Input: part model. Units: mm. Frame: model coordinates. Coordinates: 2 decimals unless noted, no trailing zeros. Use CSV: the item, a comma, the result in double quotes.
```python
from build123d import *

# Parameters (mm, degrees)
F0_R     = 19.05
F1_DEPTH = 6.35
F2_D     = 6.7564
F2_DEPTH = 6.35
F2_TIP   = 2.0298273432


# Not quite as in the source:
# - ends of sketch curves that miss each other by under 0.0002 mm in the source are joined


with BuildPart() as f1:
    # F0 (on Front) → F1 (new body)
    with BuildSketch(Plane.XZ):
        Polygon((56.0273340809, 601.6124832813), (-553.5726659191, 601.6124832813), (-553.5710625288, 576.2108431508), (-578.9710624604, 576.2111164925), (-578.9710624604, -33.3878754139), (-553.5291783666, -33.3855858849), (-553.5726659191, -58.7875167187), (56.0273340809, -58.7875167187), (56.0289342467, -33.4404784252), (81.4289375396, -33.4404784254), (81.4289375396, 576.2111164925), (55.7141526242, 576.2144141151), align=None)
        with Locations((-248.9779856181, 271.4144141151)):
            Circle(F0_R, mode=Mode.SUBTRACT)
    extrude(amount=F1_DEPTH)

    # F2
    with Locations(Plane(origin=(0, 0, 0), x_dir=(1, 0, 0), z_dir=(0, 1, 0))):
        with Locations((-477.4505604353, -588.9118862284), (-401.2505604353, -588.8575930831), (-325.0505604353, -588.9123327142), (-248.8505604357, -588.9125559571), (-172.6505604357, -588.9127792), (-96.4505604357, -588.8575930831), (-20.2505604357, -588.9132256859), (68.5912178787, -500.010992039), (68.7289375396, -423.8111164925), (68.6305625245, -347.6111164925), (68.72896387, -271.4111800281), (68.6699071802, -195.2112029133), (68.7289375396, -119.0112029133), (68.7092518575, -42.8112054561), (-20.1613931545, 46.0873960761), (-96.3613931545, 46.0875217216), (-172.5613931536, 46.0871547073), (-248.7613931536, 46.0870340229), (-324.9613931536, 46.0869133385), (-401.1613931536, 46.0875167187), (-477.3613931536, 46.0866719696), (-566.2527381441, -42.8121245861), (-566.2710624604, -119.0121245861), (-566.2579736841, -195.2121245861), (-566.260591454, -271.4121245861), (-566.263209224, -347.6121245861), (-566.3166356603, -423.8121062841), (-566.2684447633, -500.0121062841)):
            Hole(F2_D / 2, depth=F2_DEPTH)
            with Locations((0, 0, -(F2_DEPTH + F2_TIP / 2))):  # 118° drill point
                Cone(0, F2_D / 2, F2_TIP, mode=Mode.SUBTRACT)


solid = f1.part
```
(1) Draft query along Z for faces 1 (the cylindrical face through (-230.81, -3.13, 277.14)), 2 (the flat face through (-327, -6.35, 276)). Return one class per face: pulls with the +Z half, pulls with the -Z half, needs draft (parallel to the pull), parting line crosses it, or undercut.
Check values:
face 1,"undercut"
face 2,"needs draft"
(2) Ray query, probe 1 along Z at (x, y) = (-325, -5.25); probe 2 along Z at (x, y) = (-403, -4.75); probe 3 along Z at (x, y) = (-239, -4.5). Return the intervals inside material, ascending. Write a range as from..to.
Check values:
probe 1,"-58.79..-49.46, -42.71..585.53, 592.29..601.61"
probe 2,"-58.79..-48.92, -43.25..585.97, 591.75..601.61"
probe 3,"-58.79..255.19, 287.64..601.61"
(3) Pin query (flat end, axial travel): pin 1 Ø4 at (x, z) = (68.73, 119.01) entering from -Y. Return the tip coordinate at first contact, or that it passes through.
Check values:
pin 1,"through"
